```python
from build123d import *

# Parameters (mm, degrees)
SKETCH_1_R               = 20.5
SKETCH_1_R_2             = 6.5
SKETCH_1_R_3             = 1.5
EXTRUDE_1_DEPTH          = 10
SKETCH_2_R               = 4.1
CUT_EXTRUDE_1_DEPTH      = 10
SKETCH_4_W               = 41
SKETCH_4_H               = 120.125
CUT_EXTRUDE_3_DEPTH      = 5
CUT_EXTRUDE_4_DEPTH      = 195.839677684
CUT_EXTRUDE_4_DEPTH_BACK = 10
CUT_EXTRUDE_5_DEPTH      = 195.839677684
CUT_EXTRUDE_5_DEPTH_BACK = 10
SKETCH_5_R               = 1
CUT_EXTRUDE_6_DEPTH      = 195.647116598
SKETCH_6_R               = 2.5
CUT_EXTRUDE_7_DEPTH      = 10
CUT_EXTRUDE_START        = -10
SKETCH_7_R               = 5
CUT_EXTRUDE_8_DEPTH      = 1.8
FILLET_1_R               = 0.2


with BuildPart() as part:
    # 스케치1 → 보스-돌출1 (new body)
    # profile 1 of 3: a face of its own
    with BuildSketch(Plane.XY):
        with BuildLine():
            Line((-20.5, 173), (-20.5, 0))
            ThreePointArc((-20.5, 0), (0, 20.5), (20.5, 0))
            Line((20.5, 0), (20.5, 173))
            ThreePointArc((20.5, 173), (0, 152.5), (-20.5, 173))
        make_face()
    # profile 2 of 3: a face of its own
    with BuildSketch(Plane.XY):
        with Locations((0, 173)):
            Circle(SKETCH_1_R)
    # profile 3 of 3: a face of its own
    with BuildSketch(Plane.XY):
        Circle(SKETCH_1_R)
        with Locations((0, -7)):
            Circle(SKETCH_1_R_2, mode=Mode.SUBTRACT)
        with Locations((-7.75, -13.423393759)):
            Circle(SKETCH_1_R_3, mode=Mode.SUBTRACT)
        with Locations((7.75, -13.423393759)):
            Circle(SKETCH_1_R_3, mode=Mode.SUBTRACT)
        with Locations((15.5, 0)):
            Circle(SKETCH_1_R_3, mode=Mode.SUBTRACT)
        with Locations((7.75, 13.423393759)):
            Circle(SKETCH_1_R_3, mode=Mode.SUBTRACT)
        with Locations((-7.75, 13.423393759)):
            Circle(SKETCH_1_R_3, mode=Mode.SUBTRACT)
        with Locations((-15.5, 0)):
            Circle(SKETCH_1_R_3, mode=Mode.SUBTRACT)
    extrude(amount=-EXTRUDE_1_DEPTH)

    # 스케치2 → 컷-돌출1 (cut)
    with BuildSketch(Plane.XY):
        with Locations((0, 173)):
            Circle(SKETCH_2_R)
        with Locations((0, 143)):
            Circle(SKETCH_2_R)
    extrude(amount=-CUT_EXTRUDE_1_DEPTH, mode=Mode.SUBTRACT)

    # 스케치4 → 컷-돌출3 (cut)
    with BuildSketch(Plane.XY):
        with Locations((0, 39.5625)):
            Rectangle(SKETCH_4_W, SKETCH_4_H)
    extrude(amount=-CUT_EXTRUDE_3_DEPTH, mode=Mode.SUBTRACT)

    # 스케치3 → 컷-돌출4 (cut, two sides: drawn at the far end of the back side and taken through both)
    with BuildSketch(Plane.XY.offset(-CUT_EXTRUDE_4_DEPTH_BACK)):
        Polygon((15.5, 125.455788946), (3.235714571, 115.8125), (15.5, 106.169211054), align=None)
        Polygon((12.264285429, 103.625), (0, 113.268288946), (-12.264285429, 103.625), align=None)
        Polygon((-3.235714571, 115.8125), (-15.5, 125.455788946), (-15.5, 106.169211054), align=None)
    extrude(amount=CUT_EXTRUDE_4_DEPTH + CUT_EXTRUDE_4_DEPTH_BACK, mode=Mode.SUBTRACT)

    # 스케치3<4> → 컷-돌출5 (cut, two sides: drawn at the far end of the back side and taken through both)
    with BuildSketch(Plane.XY.offset(-CUT_EXTRUDE_5_DEPTH_BACK)):
        Polygon((12.830480138, 99.625), (-12.830480138, 99.625), (0, 85.112071418), align=None)
        Polygon((15.5, 67.579571418), (15.5, 96.605428582), (2.669519862, 82.0925), align=None)
        Polygon((12.830480138, 64.56), (0, 79.072928582), (-12.830480138, 64.56), align=None)
        Polygon((-2.669519862, 82.0925), (-15.5, 96.605428582), (-15.5, 67.579571418), align=None)
        Polygon((12.830313114, 60.56), (-12.830313114, 60.56), (0, 46.049329749), align=None)
        Polygon((-2.669686886, 43.03), (-15.5, 57.540670251), (-15.5, 28.519329749), align=None)
        Polygon((12.830313114, 25.5), (0, 40.010670251), (-12.830313114, 25.5), align=None)
        Polygon((15.5, 28.519329749), (15.5, 57.540670251), (2.669686886, 43.03), align=None)
    extrude(amount=CUT_EXTRUDE_5_DEPTH + CUT_EXTRUDE_5_DEPTH_BACK, mode=Mode.SUBTRACT)

    # 스케치5 → 컷-돌출6 (cut, through all)
    with BuildSketch(Plane.XY.offset(-5)):
        with Locations((-15.33, 23)):
            Circle(SKETCH_5_R)
        with Locations((-10.16, 23)):
            Circle(SKETCH_5_R)
        with Locations((10.16, 23)):
            Circle(SKETCH_5_R)
        with Locations((15.33, 23)):
            Circle(SKETCH_5_R)
        with Locations((-15.33, 62.56)):
            Circle(SKETCH_5_R)
        with Locations((-10.16, 62.56)):
            Circle(SKETCH_5_R)
        with Locations((10.16, 62.56)):
            Circle(SKETCH_5_R)
        with Locations((15.33, 62.56)):
            Circle(SKETCH_5_R)
    extrude(amount=-CUT_EXTRUDE_6_DEPTH, mode=Mode.SUBTRACT)

    # 스케치6 → 컷-돌출7 (cut)
    with BuildSketch(Plane.XY):
        with Locations((-12.37, 135.5)):
            Circle(SKETCH_6_R)
        with Locations((12.375, 135.5)):
            Circle(SKETCH_6_R)
        with Locations((0, 123)):
            Circle(SKETCH_6_R)
    extrude(amount=-CUT_EXTRUDE_7_DEPTH, mode=Mode.SUBTRACT)

    # 스케치7 → 컷-돌출8 (cut)
    with BuildSketch(Plane.XY.offset(CUT_EXTRUDE_START)):
        with Locations((0, 173)):
            Circle(SKETCH_7_R)
        with Locations((0, 143)):
            Circle(SKETCH_7_R)
    extrude(amount=CUT_EXTRUDE_8_DEPTH, mode=Mode.SUBTRACT)

    # 필렛1
    fillet_1_edges = [part.edges().sort_by_distance(p)[0] for p in [
        (-4.1, 173, -8.2),
        (-5, 173, -10),
        (-4.1, 143, -8.2),
        (-5, 143, -10),
    ]]
    fillet(fillet_1_edges, radius=FILLET_1_R)


solid = part.part
```
Source: CAD feature listing. Evaluate the final solid. Frame: model axes, mm. A direction names the side the tool comes from. Coordinates: 2 decimals unless noted, no trailing zeros. Loops run counter-clockwise (first coordinate to the right, second up) from the corner with the lowest first, then second, coordinate; pieces in that order, holes last. Notation, with made-up numbers: M 81.5,-12.75 L 133.5,-12.75 A23 ccw 133.5,13.25 Z; hole C 36,-19.5 d1. An arc over 180 degrees is marked long. Use a Markdown table: item, result. Add a question column.
Q1. Material intervals for L1, parallel to Y at x = 16, z = -5.5; L2, parallel to Y at x = 13, z = -5.25; L3, parallel to X at y = 175.5, z = -3.5, sorted ascending.
Q2. First-contact query: pin 1 (3.5 mm diameter, centred on x = -15.5, y = 0, fed in from +Z); pin 2 (5 mm diameter, centred on x = -15.5, z = -9, fed in from +Y); pin 3 (2.5 mm diameter, centred on x = 4, z = -6.5, fed in from +Y); pin 4 (4 mm diameter, centred on x = 12.375, y = 135.5, fed in from -Z). Flat tips, straight axial feed; report the tip coordinate or a pass-through.
Q3. Access query for faces 1 (the flat face through (15.5, 116, -5)), 2 (the cylindrical face through (-0.651, 177.957, -9.011)). Directions: +Z, -Z, +X, -X, +Y, -Y. A direction counts if a zero-diameter tool reaches every point of the face in a straight line with its end or side. Return the directions, or none.
Q4. Section query A-A, the plane y = 143. Return loops of the section in (x, z).
Q5. Draft query along Y for faces 3 (the flat face through (-20.5, 107, -6)), 4 (the flat face through (-15.5, 43, -8)). Return one class per face: pulls with the +Y half, pulls with the -Y half, needs draft (parallel to the pull), parting line crosses it, or undercut.
Q6. Section query C-C, the plane y = 52. Return loops of the section in (x, z), and give its area (3 significant figures).
Q7. Section query D-D, the plane y = -7. Return loops of the section in (x, z).
Q8. Section query B-B, the plane z = -1.5. State how many separate pieces and enclosed holes the cut face has, and give its area (3 significant figures).
Result:
| question | item | result |
|---|---|---|
| 1 | L1 | y = -12.82 to -1.41, 1.41 to 22.26, 23.74 to 61.82, 63.3 to 185.82 |
| 1 | L2 | y = -15.85 to 31.35, 54.71 to 70.41, 93.78 to 108.13, 123.49 to 133.08, 137.92 to 188.85 |
| 1 | L3 | x = -20.35 to -3.25, 3.25 to 20.35 |
| 2 | pin 1 | stops at z = -5 |
| 2 | pin 2 | stops at y = 188.85 |
| 2 | pin 3 | stops at y = 193.31 |
| 2 | pin 4 | passes through |
| 3 | face 1 | +Z, -Z |
| 3 | face 2 | -Z |
| 4 | outline | M -20.5,-10 L -5.2,-10 A0.2 ccw -5,-9.8 L -5,-8.2 L -4.3,-8.2 A0.2 ccw -4.1,-8 L -4.1,0 L -20.5,0 Z; M 4.1,-8 A0.2 ccw 4.3,-8.2 L 5,-8.2 L 5,-9.8 A0.2 ccw 5.2,-10 L 20.5,-10 L 20.5,0 L 4.1,0 Z |
| 5 | face 3 | needs draft |
| 5 | face 4 | undercut |
| 6 | outline | M -20.5,-10 L -15.5,-10 L -15.5,-5 L -20.5,-5 Z; M -10.6,-10 L -5.26,-10 L -5.26,-5 L -10.6,-5 Z; M 5.26,-10 L 10.6,-10 L 10.6,-5 L 5.26,-5 Z; M 15.5,-10 L 20.5,-10 L 20.5,-5 L 15.5,-5 Z |
| 6 | area | 103 mm2 |
| 7 | outline | M -19.27,-10 L -6.5,-10 L -6.5,-5 L -19.27,-5 Z; M 6.5,-10 L 19.27,-10 L 19.27,-5 L 6.5,-5 Z |
| 8 | separate pieces | 1 |
| 8 | enclosed holes | 8 |
| 8 | area | 3,150 mm2 |
